Geometry: see drawing. Coordinates: mm, zero at the bounding-box minimum. A direction names the side the tool comes from. Round coordinates to 2 decimals unless told otherwise and drop trailing zeros. Order: outer loops, then holes, each group sorted by start corner. A loop starts at its lowest first (then second) coordinate and runs counter-clockwise, first axis right, second up. Notation, with made-up numbers: (-7.5, -25.5) -> (29.5, -25.5) arc R35 ccw to (29.5, 6.5) -> close; hole circle Ø2 at (43.25, 75.25). An arc over 180 degrees is marked (long way). One line per item, written item: value. Start each with the question number.
1) Section C-C (z = 13.75). Return the cut outline in (x, y) (1 decimal), and give its area (3 significant figures).
2) Mould query, pull axis X, two halves, no side actions, for the marked faces 1, 2, 3 and 4. Classes: pulls with the +X half, pulls with the -X half, needs draft (parallel to the pull), parting line crosses it, or undercut.
3) Section A-A (y = 7). Return the cut outline in (x, z), and give its area (3 significant figures).
4) Ray query, L1, parallel to X at y = 70.5, z = 3.25 (1 decimal); L2, parallel to Y at x = 117, z = 1.5; L3, parallel to Y at x = 73.5, z = 14.75 (1 decimal). Return the intervals inside material, ascending.
5) Pin query (flat end, axial travel): P1, Ø17, axis at x = 115.66, y = 21.59, coming from the +Z side; P2, Ø3, axis at y = 51, z = 21, coming from the -X side; P3, Ø25, axis at x = 78, y = 47.5, coming from the -Z side (1 decimal). Return the tip coordinate at first contact, or that it passes through.
6) Section B-B (x = 112). Return the cut outline in (y, z), and give its area (3 significant figures).
7) Section D-D (y = 70.5). Return the cut outline in (x, z) (1 decimal), and give its area (3 significant figures).
8) Reachability of the marked faces 5, 6 and 7 from +Z, -Z, +X, -X, +Y, -Y: full face, straight path, thin tool, end or side. Return the list, or none.
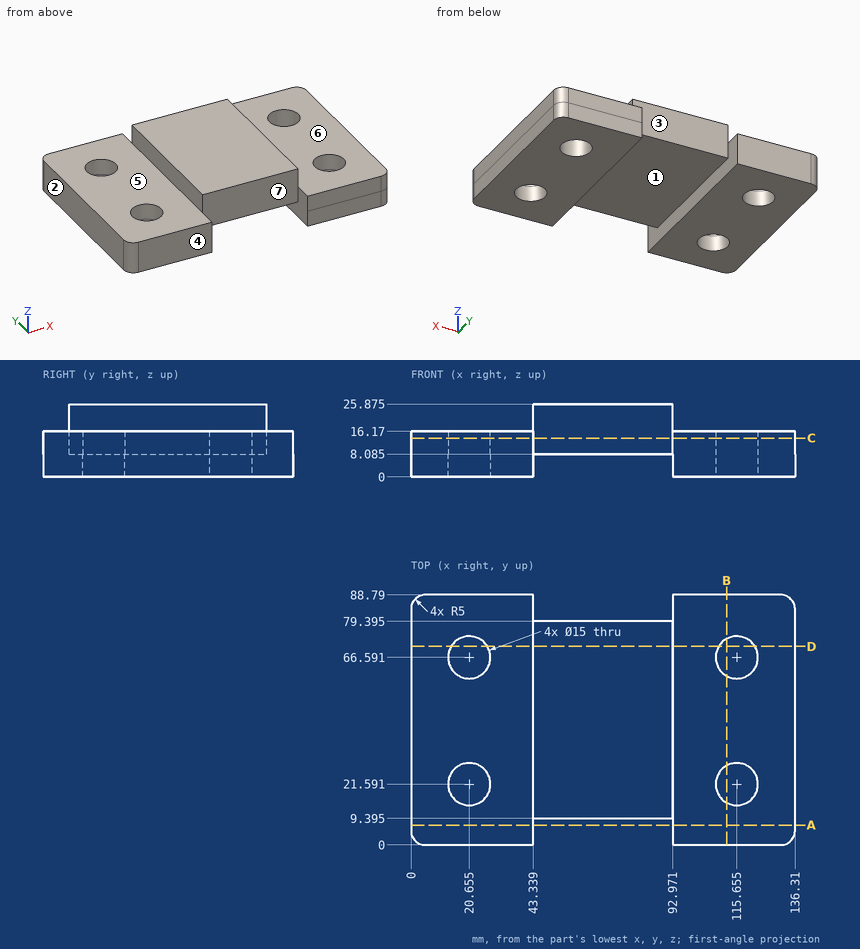
Findings:
1. outline: (0, 5) arc R5 ccw to (5, 0) -> (43.3, 0) -> (43.3, 9.4) -> (93, 9.4) -> (93, 0) -> (131.3, 0) arc R5 ccw to (136.3, 5) -> (136.3, 83.8) arc R5 ccw to (131.3, 88.8) -> (93, 88.8) -> (93, 79.4) -> (43.3, 79.4) -> (43.3, 88.8) -> (5, 88.8) arc R5 ccw to (0, 83.8) -> close; hole circle Ø15 at (20.7, 21.6); hole circle Ø15 at (20.7, 66.6); hole circle Ø15 at (115.7, 21.6); hole circle Ø15 at (115.7, 66.6)
1. area: 10,400 mm2
2. face 1: undercut
2. face 2: pulls with the -X half
2. face 3: undercut
2. face 4: needs draft
3. outline: (0, 0) -> (43.34, 0) -> (43.34, 16.17) -> (0, 16.17) -> close; (92.97, 0) -> (136.31, 0) -> (136.31, 16.17) -> (92.97, 16.17) -> close
3. area: 1,400 mm2
4. L1: 0 to 14.3, 27.1 to 43.3, 93 to 109.3, 122.1 to 136.3
4. L2: 0 to 14.21, 28.97 to 59.21, 73.97 to 88.79
4. L3: 9.4 to 79.4
5. P1: z = 16.17
5. P2: x = 43.34
5. P3: z = 8.1
6. outline: (0, 0) -> (15.04, 0) -> (15.04, 16.17) -> (0, 16.17) -> close; (28.14, 0) -> (60.04, 0) -> (60.04, 16.17) -> (28.14, 16.17) -> close; (73.14, 0) -> (88.79, 0) -> (88.79, 16.17) -> (73.14, 16.17) -> close
6. area: 1,010 mm2
7. outline: (0, 0) -> (14.3, 0) -> (14.3, 16.2) -> (0, 16.2) -> close; (27.1, 0) -> (43.3, 0) -> (43.3, 8.1) -> (93, 8.1) -> (93, 0) -> (109.3, 0) -> (109.3, 16.2) -> (93, 16.2) -> (93, 25.9) -> (43.3, 25.9) -> (43.3, 16.2) -> (27.1, 16.2) -> close; (122.1, 0) -> (136.3, 0) -> (136.3, 16.2) -> (122.1, 16.2) -> close
7. area: 1,870 mm2
8. face 5: +Z, -X, +Y, -Y
8. face 6: +Z, +X, +Y, -Y
8. face 7: +Z, -Z, -Y
